```python
from build123d import *

# Parameters (mm, degrees)
CUT_EXTRUDE1_DEPTH = 12
CUT_EXTRUDE2_START = -4
SKETCH4_R          = 2
CUT_EXTRUDE2_DEPTH = 4


with BuildPart() as part:
    # Sketch1 → Revolve1 (revolve)
    with BuildSketch(Plane(origin=(0, 0, 0), x_dir=(0, 0, -1), z_dir=(1, 0, 0)), mode=Mode.PRIVATE) as revolve1_sk:
        Polygon((-8, 0), (8, 0), (8, 12), (7, 12), (4.5, 6), (2, 6), (0.2, 12), (-0.2, 12), (-2, 6), (-4.5, 6), (-7, 12), (-8, 12), align=None)
    revolve(revolve1_sk.sketch.rotate(Axis((0, 0, 8), (0, 0, -1)), 90), axis=Axis((0, 0, 8), (0, 0, -1)))

    # Sketch3 → Cut-Extrude1 (cut)
    with BuildSketch(Plane(origin=(0, 0, -8), x_dir=(-1, 0, 0), z_dir=(0, 0, -1))):
        with BuildLine():
            Line((-1.322875656, 1.5), (1.322875656, 1.5))
            ThreePointArc((1.322875656, 1.5), (0, -2), (-1.322875656, 1.5))
        make_face()
    extrude(amount=-CUT_EXTRUDE1_DEPTH, mode=Mode.SUBTRACT)

    # Sketch4 → Cut-Extrude2 (cut)
    with BuildSketch(Plane.XY.offset(8).offset(CUT_EXTRUDE2_START)):
        with Locations(Location((0, 0, 0), (0, 0, 131.409622109))):
            Circle(SKETCH4_R)
    extrude(amount=CUT_EXTRUDE2_DEPTH, mode=Mode.SUBTRACT)


solid = part.part
```
Check sheet for the modelled part. Datum: model origin and axes. Units: mm. A direction names the side the tool comes from. Give positions to 0.01 mm unless a question says otherwise; leave off trailing zeros. Order: outer loops, then holes, each group sorted by start corner. A loop starts at its lowest first (then second) coordinate and runs counter-clockwise, first axis right, second up. Notation, with made-up numbers: M -18.75,-2.5 L -5.75,-2.5 A22 cw -5.75,9.5 Z; hole C 6,-21.75 d4. An arc over 180 degrees is marked long. Answer in a Markdown table with one row per item.
1) Cross-section at D-D, the plane z = -2.5. Enter the section's corners in (x, y).
Filled sheet:
| item | result |
|---|---|
| outline | C 0,0 d12; hole M -1.32,1.5 A2 ccw long 1.32,1.5 Z |
2) Cross-section at C-C, the plane y = -10.25. Count the separate pieces of the cut face and the enclosed holes in it, plus the area to 3 significant figures.
Filled sheet:
| item | result |
|---|---|
| separate pieces | 3 |
| enclosed holes | 0 |
| area | 50.5 mm2 |
3) Cross-section at B-B, the plane x = 0. Enter the section's corners in (y, z), plus the area to 3 significant figures.
Filled sheet:
| item | result |
|---|---|
| outline | M -12,-8 L -2,-8 L -2,8 L -12,8 L -12,7 L -6,4.5 L -6,2 L -12,0.2 L -12,-0.2 L -6,-2 L -6,-4.5 L -12,-7 Z; M 1.5,-8 L 12,-8 L 12,-7 L 6,-4.5 L 6,-2 L 12,-0.2 L 12,0.2 L 6,2 L 6,4.5 L 12,7 L 12,8 L 2,8 L 2,4 L 1.5,4 Z |
| area | 214 mm2 |
4) Thickness scan on L1, parallel to Z at x = -2.5, y = -6.25; L2, parallel to Z at x = -3, y = 10.5; L3, parallel to Y at x = 0, z = 6.2. Record the ranges inside material, lowest first. Write a range as [from, to].
Filled sheet:
| item | result |
|---|---|
| L1 | z = [-8, -4.8], [-1.78, 1.78], [4.8, 8] |
| L2 | z = [-8, -6.55], [-0.52, 0.52], [6.55, 8] |
| L3 | y = [-10.08, -2], [2, 10.08] |
5) Release check for a two-part mould opening along X. For faces 3 (the flat face through (0, 1.5, -2)), 4 (the flat face through (-2.5, -0.2, -8)), 5 (the conical face through (-1.36, 6.14, -4.62)) record: +X half, -X half, draft (parallel to the pull), parting line (faces both ways), or undercut.
Filled sheet:
| item | result |
|---|---|
| face 3 | undercut |
| face 4 | draft |
| face 5 | parting line |
6) Access from +Z, -Z, +X, -X, +Y, -Y to the whole of each face (thin tool, end or side, straight path). Record for faces 1 (the cylindrical face through (11.446, -3.604, 0.003)), 2 (the cylindrical face through (5.723, -1.802, -3.232)).
Filled sheet:
| item | result |
|---|---|
| face 1 | +Z, -Z |
| face 2 | none |
7) Cross-section at A-A, the plane y = 0. Enter the section's corners in (x, z).
Filled sheet:
| item | result |
|---|---|
| outline | M -12,-8 L -2,-8 L -2,8 L -12,8 L -12,7 L -6,4.5 L -6,2 L -12,0.2 L -12,-0.2 L -6,-2 L -6,-4.5 L -12,-7 Z; M 2,-8 L 12,-8 L 12,-7 L 6,-4.5 L 6,-2 L 12,-0.2 L 12,0.2 L 6,2 L 6,4.5 L 12,7 L 12,8 L 2,8 Z |
8) Gauge pin test, flat ends, axial feed: P1, Ø1, axis at y = -5, z = -0.5, coming from the -X side; P2, Ø1, axis at x = -1.5, z = 4.5, coming from the +Y side; P3, Ø2.5, axis at x = 0, y = 0, coming from the +Z side; P4, Ø1.3, axis at x = 0.5, z = -4.5, coming from the -Y side. Record the tip position at first contact, or that the pin passes through.
Filled sheet:
| item | result |
|---|---|
| P1 | stops at x = -11.08 |
| P2 | stops at y = 7.05 |
| P3 | passes through |
| P4 | stops at y = -7.54 |
